Source: CAD feature listing. Evaluate the final solid. Frame: model axes, mm. Round coordinates to 2 decimals unless told otherwise and drop trailing zeros. Order: outer loops, then holes, each group sorted by start corner. A loop starts at its lowest first (then second) coordinate and runs counter-clockwise, first axis right, second up. Notation, with made-up numbers: (20.5, 38.5) - (24.5, 38.5) arc R26 ccw to (24.5, 68.5) - close; hole circle Ø2 at (-35, 31). An arc over 180 degrees is marked (long way). Put each result on its own line as item: value. Start each with the question number.
1) Section C-C on y = -10.75. Output: boundary loops of the cut face in (x, z), then the cut area to 3 significant figures.
2) Section A-A on x = 0. Output: boundary loops of the cut face in (y, z).
3) Line query: probe 1 along Y at (x, z) = (0, 8); probe 2 along X at (y, z) = (-10, -12); probe 3 along X at (y, z) = (-10, 22). Output: solid intervals per line, ascending. Write a range as [from, to].
4) Section B-B on z = -2. Output: boundary loops of the cut face in (x, y).
5) Section D-D on y = -15.5. Output: boundary loops of the cut face in (x, z), then the cut area to 3 significant figures.
6) Contact query for flat-ended pins moving along their axis: P1, Ø3, axis at y = -8, z = -20, coming from the +X side; P2, Ø8, axis at x = 16.5, y = -16.5, coming from the -Z side; P3, Ø6, axis at x = -10, y = -14.5, coming from the +Z side. Output: stop coordinate, or through.
```python
from build123d import *

# Parameters (mm, degrees)
F0_R     = 28.5
F1_DEPTH = 20
F2_R     = 4
F3_DEPTH = 28.501
F4_DEPTH = 28.501


with BuildPart() as f1:
    # F0 (on Front) → F1 (new body)
    with BuildSketch(Plane.XZ):
        Circle(F0_R)
    extrude(amount=F1_DEPTH)

    # F2 (on Top) → F3 (cut, through all)
    with BuildSketch(Plane.XY):
        with Locations((0, -10)):
            Circle(F2_R)
    extrude(amount=-F3_DEPTH, mode=Mode.SUBTRACT)

    # F2 (on Top) → F4 (cut, through all)
    with BuildSketch(Plane.XY):
        with Locations((0, -10)):
            Circle(F2_R)
    extrude(amount=F4_DEPTH, mode=Mode.SUBTRACT)


solid = f1.part
```
Answer sheet:
1. outline: (-3.93, -28.23) - (-3.93, 28.23) arc R28.5 ccw to start; (3.93, -28.23) arc R28.5 ccw to (3.93, 28.23) - close
1. area: 2,110 mm^2
2. outline: (-20, -28.5) - (-14, -28.5) - (-14, 28.5) - (-20, 28.5) - close; (-6, -28.5) - (0, -28.5) - (0, 28.5) - (-6, 28.5) - close
3. probe 1: [-20, -14], [-6, 0]
3. probe 2: [-25.85, -4], [4, 25.85]
3. probe 3: [-18.12, -4], [4, 18.12]
4. outline: (-28.43, -20) - (28.43, -20) - (28.43, 0) - (-28.43, 0) - close; hole circle Ø8 at (0, -10)
5. outline: circle Ø57 at (0, 0)
5. area: 2,550 mm^2
6. P1: x = 21.68
6. P2: z = -25.61
6. P3: z = 27.63
